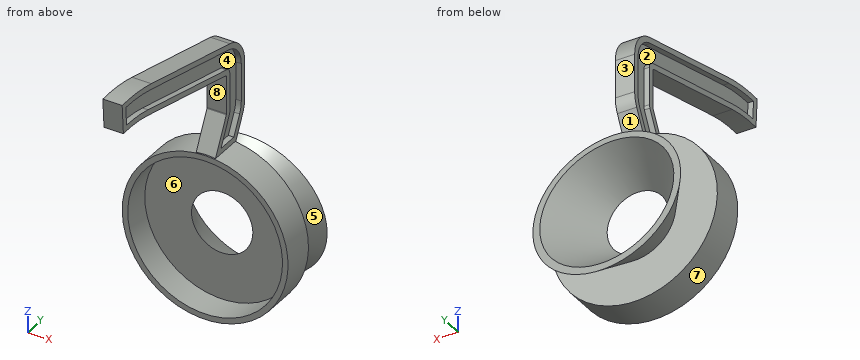
from build123d import *

# Parameters (mm, degrees)
SWEEP2_START       = -8.89
SWEEP2_DEPTH       = 17.78
FILLET1_R          = 28.448
FILLET2_R          = 1.524
CUT_EXTRUDE1_DEPTH = 5.08


with BuildPart() as part:
    # Sketch1 → Revolve1 (revolve)
    with BuildSketch(Plane.XY, mode=Mode.PRIVATE) as revolve1_sk:
        Polygon((71.12, 25.4), (28.194, 25.4), (68.685755738, 81.378294554), (75.018953762, 81.51903327), (38.1, 30.48), (76.2, 30.48), (76.2, 0), (71.12, 0), align=None)
    revolve(revolve1_sk.sketch.rotate(Axis((0, 85.716301318, 0), (0, -1, 0)), 90), axis=Axis((0, 85.716301318, 0), (0, -1, 0)))

    # SurfaceCut1
    split(bisect_by=Plane(origin=(0, 69.471471591, 9.763578605), x_dir=(-1, 0, 0), z_dir=(0, 0.9902680687415703, 0.13917310096006574)), keep=Keep.BOTTOM)

    # Sweep2: read off the stored shape, not the designer's step
    # Sweep2 outline → Sweep2 (add)
    with BuildSketch(Plane.YZ.offset(SWEEP2_START)):
        with BuildLine():
            Line((17.370160471, 143.002), (17.370160471, 107.987503449))
            Line((17.370160471, 107.987503449), (1.021963911, 75.67963993))
            Line((1.021963911, 75.67963993), (30.48, 75.67963993))
            Line((30.48, 75.67963993), (30.48, 73.66))
            Line((30.48, 73.66), (44.566575341, 101.498370543))
            Line((44.566575341, 101.498370543), (44.566575341, 143.002))
            ThreePointArc((44.566575341, 143.002), (38.336028216, 160.835083682), (22.355619148, 170.908073165))
            Line((22.355619148, 170.908073165), (-94.754140244, 197.729788602))
            ThreePointArc((-94.754140244, 197.729788602), (-116.352888931, 201.043440298), (-138.203933305, 201.177947268))
            Line((-138.203933305, 201.177947268), (-136.414333354, 174.040476608))
            ThreePointArc((-136.414333354, 174.040476608), (-118.532403269, 173.934498987), (-100.856344498, 171.226806034))
            Line((-100.856344498, 171.226806034), (16.253414894, 144.405090597))
            ThreePointArc((16.253414894, 144.405090597), (17.056894537, 143.898630346), (17.370160471, 143.002))
        make_face()
    extrude(amount=SWEEP2_DEPTH)

    # Fillet1
    fillet1_edges = [part.edges().sort_by_distance(p)[0] for p in [
        (0, 44.566575341, 101.498370543),
    ]]
    fillet(fillet1_edges, radius=FILLET1_R)

    # Fillet2
    fillet2_edges = [part.edges().sort_by_distance(p)[0] for p in [
        (0, 17.370160471, 107.987503449),
    ]]
    fillet(fillet2_edges, radius=FILLET2_R)

    # Sketch7 → Cut-Extrude1 (cut)
    with BuildSketch(Plane(origin=(8.89, 0, 0), x_dir=(0, 0, -1), z_dir=(1, 0, 0))):
        with BuildLine():
            Line((-80.75963993, 9.28584823), (-80.75963993, 28.379170924))
            Line((-80.75963993, 28.379170924), (-97.73546941, 36.969160074))
            ThreePointArc((-97.73546941, 36.969160074), (-102.862715222, 38.848510317), (-108.286134805, 39.486575341))
            Line((-108.286134805, 39.486575341), (-143.002, 39.486575341))
            ThreePointArc((-143.002, 39.486575341), (-157.670443725, 34.362181678), (-165.956972893, 21.218510727))
            Line((-165.956972893, 21.218510727), (-192.778140508, -95.888856575))
            ThreePointArc((-192.778140508, -95.888856575), (-195.756406443, -114.226762874), (-196.359610136, -132.795150546))
            Line((-196.359610136, -132.795150546), (-179.348953739, -131.673370618))
            ThreePointArc((-179.348953739, -131.673370618), (-178.772717763, -115.597689457), (-176.178592901, -99.722233909))
            Line((-176.178592901, -99.722233909), (-149.355564845, 17.393241513))
            ThreePointArc((-149.355564845, 17.393241513), (-147.062179047, 21.031609572), (-143.002, 22.450160471))
            Line((-143.002, 22.450160471), (-108.351133677, 22.450160471))
            ThreePointArc((-108.351133677, 22.450160471), (-106.818428143, 22.269837747), (-105.369423892, 21.738717026))
            Line((-105.369423892, 21.738717026), (-80.75963993, 9.28584823))
        make_face()
    cut_extrude1 = extrude(amount=-CUT_EXTRUDE1_DEPTH, mode=Mode.SUBTRACT)

    # Mirror2: Cut-Extrude1 across plane
    add(cut_extrude1.mirror(Plane(origin=(0, 0, 0), x_dir=(0, 0, 1), z_dir=(1, 0, 0))), mode=Mode.SUBTRACT)


solid = part.part
Verification items for the finished model (mm, model axes). Face numbers are marked on the shaded views. A direction names the side the tool comes from. Coordinates: 2 decimals unless noted, no trailing zeros. Order: outer loops, then holes, each group sorted by start corner. A loop starts at its lowest first (then second) coordinate and runs counter-clockwise, first axis right, second up. Notation, with made-up numbers: M 40.25,-21 L 82.25,-21 A29 ccw 82.25,18 Z; hole C -12.5,35.25 d11. An arc over 180 degrees is marked long. Write each question's results on one line, items separated by ' | '.
1) Access from +Z, -Z, +X, -X, +Y, -Y to the whole of each face (thin tool, end or side, straight path). Record for the marked faces 1, 2, 3, 4 and 5.
Solved:
face 1: +X, -X, +Y | face 2: -X | face 3: +Z, +X, -X, +Y | face 4: +X | face 5: none
2) Gauge pin test, flat ends, axial feed: pin 1 Ø5.5 at (x, z) = (7.5, 122) entering from -Y; pin 2 Ø8 at (x, z) = (-4.5, 30) entering from +Y; pin 3 Ø1.5 at (x, z) = (-7, 126) entering from +Y. Record the tip position at first contact, or that the pin passes through.
Solved:
pin 1: stops at y = 17.37 | pin 2: stops at y = 33.89 | pin 3: stops at y = 44.57
3) Section check D-D on z = 68. Record the cut outline in (x, y).
Solved:
outline: M -34.39,0 L -20.83,0 L -20.83,25.4 L 20.83,25.4 L 20.83,0 L 34.39,0 L 34.39,30.48 L -34.39,30.48 Z
4) Scan lines: line 1 along X through (y, z) = (18, 0); line 2 along Y through (x, z) = (42, -47); line 3 along Y through (x, z) = (-48.5, 0.5). Record each from-to range of solid material in increasing order. Write a range as [from, to].
Solved:
line 1: x = [-76.2, -71.12], [71.12, 76.2] | line 2: y = [25.4, 30.48], [64.95, 73.56] | line 3: y = [25.4, 30.48], [44.86, 53.48]
5) Section check A-A on z = 0. Record the cut outline in (x, y).
Solved:
outline: M -76.2,0 L -71.12,0 L -71.12,25.4 L -28.19,25.4 L -61.07,70.84 L -67.3,70.84 L -38.1,30.48 L -76.2,30.48 Z; M 28.19,25.4 L 71.12,25.4 L 71.12,0 L 76.2,0 L 76.2,30.48 L 38.1,30.48 L 67.3,70.84 L 61.07,70.84 Z
6) Section check B-B on y = 12.5. Record the cut outline in (x, z).
Solved:
outline: M -8.89,75.68 A76.2 ccw long 8.89,75.68 L 8.89,80.76 L 3.81,80.76 L 3.81,87.11 L 8.89,87.11 L 8.89,98.36 L -8.89,98.36 L -8.89,87.11 L -3.81,87.11 L -3.81,80.76 L -8.89,80.76 Z; M -8.89,145.26 L 8.89,145.26 L 8.89,150.48 L 3.81,150.48 L 3.81,167.95 L 8.89,167.95 L 8.89,173.17 L -8.89,173.17 L -8.89,167.95 L -3.81,167.95 L -3.81,150.48 L -8.89,150.48 Z; hole C 0,0 d142.24
7) Release check for a two-part mould opening along X. For the marked faces 6, 7 and 8 record: pulls with the +X half, pulls with the -X half, needs draft (parallel to the pull), parting line crosses it, or undercut.
Solved:
face 6: undercut | face 7: parting line crosses it | face 8: needs draft
